Could you check a few things on this drawing? It's one solid part, dimensions in mm from its lowest x, y, z. Round coordinates to 2 decimals unless told otherwise and drop trailing zeros. Loops run counter-clockwise (first coordinate to the right, second up) from the corner with the lowest first, then second, coordinate; pieces in that order, holes last. Notation, with made-up numbers: (-12, 18.5) -> (44, 18.5) arc R30 cw to (44, 48.5) -> close; hole circle Ø2 at (-26, 76.5). An arc over 180 degrees is marked (long way). Use one line per item in the form item = value. Start each with the question number.
Item 1: I'm going to push flat-ended pins straight in: pin 1 Ø3 at (y, z) = (3, 343) entering from +X; pin 2 Ø3 at (y, z) = (2.5, 2) entering from -X; pin 3 Ø25 at (x, z) = (245, 385) entering from +Y; pin 4 Ø1 at (x, y) = (71.5, 1.5) entering from +Z. Where does each tip first touch, or does it pass through?
Item 2: If we section it at C-C (y = 4.15): State how many separate pieces and enclosed holes the cut face has, then the cut area to 3 significant figures.
Item 3: If I drill on L1, parallel to X at y = 4, z = 315; L2, parallel to X at y = 4.25, z = 221; L3, parallel to X at y = 3.05, z = 376, over which ranges is the centre line in solid material (lowest first)? Write a range as [from, to].
Item 4: If we section it at D-D (z = 320.5): Write out the boundary of the cut face in (x, y).
Item 5: If we section it at B-B (z = 35): Write out the boundary of the cut face in (x, y), then the cut area to 3 significant figures.
Item 6: If we section it at A-A (x = 175): Write out the boundary of the cut face in (y, z), then the cut area to 3 significant figures.
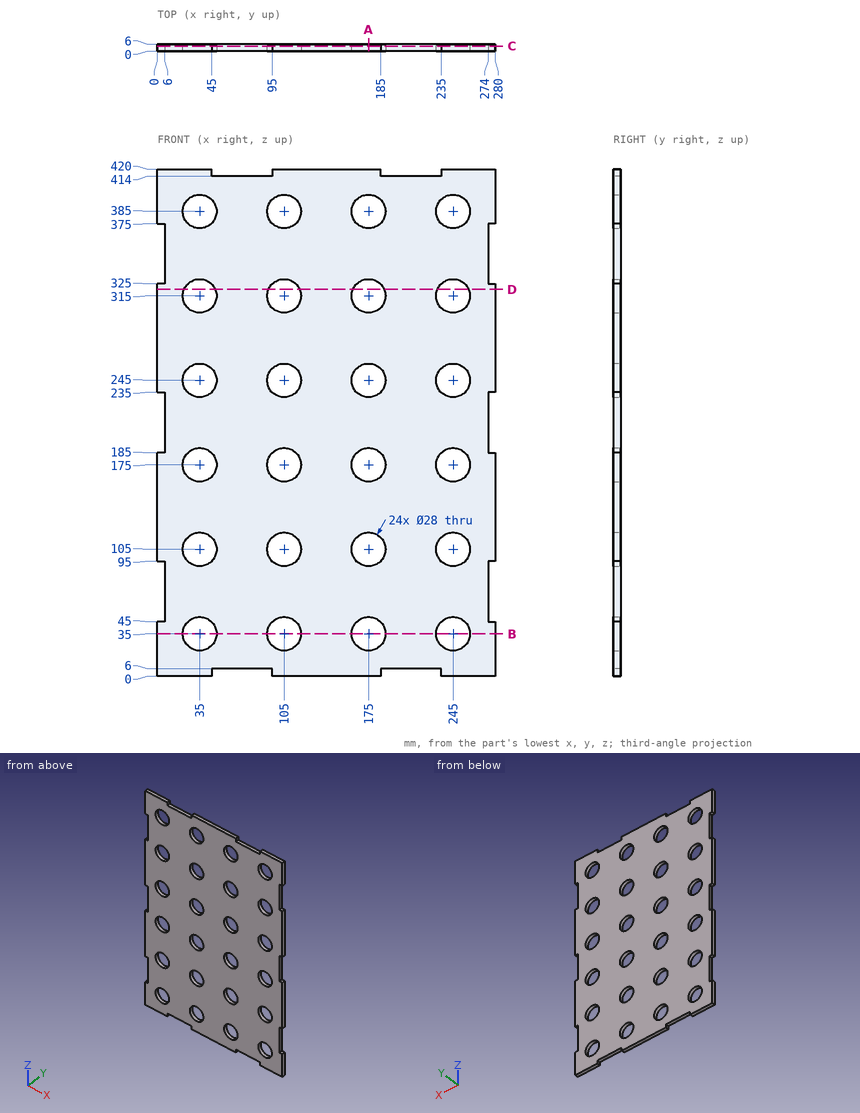
Values found:
q1.pin_1 = 274
q1.pin_2 = 0
q1.pin_3 = through
q1.pin_4 = 414
q2.separate_pieces = 1
q2.enclosed_holes = 24
q2.area = 99,800 mm2
q3.L1 = [0, 21], [49, 91], [119, 161], [189, 231], [259, 280]
q3.L2 = [6, 274]
q3.L3 = [0, 24.28], [45.72, 94.28], [115.72, 164.28], [185.72, 234.28], [255.72, 280]
q4.outline = (0, 0) -> (22.13, 0) -> (22.13, 6) -> (0, 6) -> close; (47.87, 0) -> (92.13, 0) -> (92.13, 6) -> (47.87, 6) -> close; (117.87, 0) -> (162.13, 0) -> (162.13, 6) -> (117.87, 6) -> close; (187.87, 0) -> (232.13, 0) -> (232.13, 6) -> (187.87, 6) -> close; (257.87, 0) -> (280, 0) -> (280, 6) -> (257.87, 6) -> close
q5.outline = (0, 0) -> (21, 0) -> (21, 6) -> (0, 6) -> close; (49, 0) -> (91, 0) -> (91, 6) -> (49, 6) -> close; (119, 0) -> (161, 0) -> (161, 6) -> (119, 6) -> close; (189, 0) -> (231, 0) -> (231, 6) -> (189, 6) -> close; (259, 0) -> (280, 0) -> (280, 6) -> (259, 6) -> close
q5.area = 1,010 mm2
q6.outline = (0, 0) -> (6, 0) -> (6, 21) -> (0, 21) -> close; (0, 49) -> (6, 49) -> (6, 91) -> (0, 91) -> close; (0, 119) -> (6, 119) -> (6, 161) -> (0, 161) -> close; (0, 189) -> (6, 189) -> (6, 231) -> (0, 231) -> close; (0, 259) -> (6, 259) -> (6, 301) -> (0, 301) -> close; (0, 329) -> (6, 329) -> (6, 371) -> (0, 371) -> close; (0, 399) -> (6, 399) -> (6, 420) -> (0, 420) -> close
q6.area = 1,510 mm2
